from build123d import *

# Parameters (mm, degrees)
SKETCH_1_R               = 9
SKETCH_1_R_2             = 29.6
SKETCH_1_R_3             = 1.5
EXTRUDE_1_DEPTH          = 3
CUT_EXTRUDE_1_DEPTH      = 287.481238478
CUT_EXTRUDE_1_DEPTH_BACK = 287.481238478
SKETCH_2_R               = 1.25
CUT_EXTRUDE_2_DEPTH      = 287.481238478
CUT_EXTRUDE_2_DEPTH_BACK = 287.481238478
CUT_EXTRUDE_3_DEPTH      = 287.481238478
CUT_EXTRUDE_3_DEPTH_BACK = 287.481238478
SKETCH_4_R               = 1.5


with BuildPart() as part:
    # 草图1 → 凸台-拉伸1 (new body)
    with BuildSketch(Plane(origin=(0, 0, 0), x_dir=(1, 0, 0), z_dir=(0, 1, 0))):
        with BuildLine():
            Line((71.271215686, 30), (163.728784314, 30))
            ThreePointArc((163.728784314, 30), (189.096168452, 33.068787794), (213, 42.09809972))
            ThreePointArc((213, 42.09809972), (282.5, 0), (213, -42.09809972))
            ThreePointArc((213, -42.09809972), (189.096168452, -33.068787794), (163.728784314, -30))
            Line((163.728784314, -30), (71.271215686, -30))
            ThreePointArc((71.271215686, -30), (45.903831548, -33.068787794), (22, -42.09809972))
            ThreePointArc((22, -42.09809972), (-47.5, 0), (22, 42.09809972))
            ThreePointArc((22, 42.09809972), (45.903831548, 33.068787794), (71.271215686, 30))
        make_face()
        with Locations(Location((0, 0, 0), (0, 0, 270))):
            Circle(SKETCH_1_R, mode=Mode.SUBTRACT)
        with Locations(Location((235, 0, 0), (0, 0, 270))):
            Circle(SKETCH_1_R_2, mode=Mode.SUBTRACT)
        with Locations(Location((218.735954124, 39.264880132, 0), (0, 0, 270))):
            Circle(SKETCH_1_R_3, mode=Mode.SUBTRACT)
        with Locations(Location((251.264045876, 39.264880132, 0), (0, 0, 270))):
            Circle(SKETCH_1_R_3, mode=Mode.SUBTRACT)
        with Locations(Location((274.264880132, 16.264045876, 0), (0, 0, 270))):
            Circle(SKETCH_1_R_3, mode=Mode.SUBTRACT)
        with Locations(Location((195.735119868, 16.264045876, 0), (0, 0, 270))):
            Circle(SKETCH_1_R_3, mode=Mode.SUBTRACT)
        with Locations(Location((195.735119868, -16.264045876, 0), (0, 0, 270))):
            Circle(SKETCH_1_R_3, mode=Mode.SUBTRACT)
        with Locations(Location((274.264880132, -16.264045876, 0), (0, 0, 270))):
            Circle(SKETCH_1_R_3, mode=Mode.SUBTRACT)
        with Locations(Location((251.264045876, -39.264880132, 0), (0, 0, 270))):
            Circle(SKETCH_1_R_3, mode=Mode.SUBTRACT)
        with Locations(Location((218.735954124, -39.264880132, 0), (0, 0, 270))):
            Circle(SKETCH_1_R_3, mode=Mode.SUBTRACT)
        with Locations(Location((-16.264045876, 39.264880132, 0), (0, 0, 270))):
            Circle(SKETCH_1_R_3, mode=Mode.SUBTRACT)
        with Locations(Location((16.264045876, 39.264880132, 0), (0, 0, 270))):
            Circle(SKETCH_1_R_3, mode=Mode.SUBTRACT)
        with Locations(Location((39.264880132, 16.264045876, 0), (0, 0, 270))):
            Circle(SKETCH_1_R_3, mode=Mode.SUBTRACT)
        with Locations(Location((39.264880132, -16.264045876, 0), (0, 0, 270))):
            Circle(SKETCH_1_R_3, mode=Mode.SUBTRACT)
        with Locations(Location((16.264045876, -39.264880132, 0), (0, 0, 270))):
            Circle(SKETCH_1_R_3, mode=Mode.SUBTRACT)
        with Locations(Location((-16.264045876, -39.264880132, 0), (0, 0, 270))):
            Circle(SKETCH_1_R_3, mode=Mode.SUBTRACT)
        with Locations(Location((-39.264880132, -16.264045876, 0), (0, 0, 270))):
            Circle(SKETCH_1_R_3, mode=Mode.SUBTRACT)
        with Locations(Location((-39.264880132, 16.264045876, 0), (0, 0, 270))):
            Circle(SKETCH_1_R_3, mode=Mode.SUBTRACT)
        with Locations(Location((-6.783865663, 11.75, 0), (0, 0, 270))):
            Circle(SKETCH_1_R_3, mode=Mode.SUBTRACT)
        with Locations(Location((6.783865663, 11.75, 0), (0, 0, 270))):
            Circle(SKETCH_1_R_3, mode=Mode.SUBTRACT)
        with Locations(Location((13.567731326, 0, 0), (0, 0, 270))):
            Circle(SKETCH_1_R_3, mode=Mode.SUBTRACT)
        with Locations(Location((6.783865663, -11.75, 0), (0, 0, 270))):
            Circle(SKETCH_1_R_3, mode=Mode.SUBTRACT)
        with Locations(Location((-13.567731326, 0, 0), (0, 0, 270))):
            Circle(SKETCH_1_R_3, mode=Mode.SUBTRACT)
        with Locations(Location((-6.783865663, -11.75, 0), (0, 0, 270))):
            Circle(SKETCH_1_R_3, mode=Mode.SUBTRACT)
    extrude(amount=EXTRUDE_1_DEPTH)

    # 草图2 → 切除-拉伸1 (cut, two sides: drawn at the far end of the back side and taken through both)
    with BuildSketch(Plane(origin=(0, 3, 0), x_dir=(1, 0, 0), z_dir=(0, 1, 0)).offset(-CUT_EXTRUDE_1_DEPTH_BACK)):
        with Locations(Location((93.271215686, 25, 0), (0, 0, 270))):
            Circle(SKETCH_2_R)
        with Locations(Location((141.728784314, 25, 0), (0, 0, 270))):
            Circle(SKETCH_2_R)
        with Locations(Location((190.288457303, 28.213023457, 0), (0, 0, 270))):
            Circle(SKETCH_2_R)
        with Locations(Location((44.711542697, 28.213023457, 0), (0, 0, 270))):
            Circle(SKETCH_2_R)
        with Locations(Location((44.711542697, -28.213023457, 0), (0, 0, 270))):
            Circle(SKETCH_2_R)
        with Locations(Location((93.271215686, -25, 0), (0, 0, 270))):
            Circle(SKETCH_2_R)
        with Locations(Location((190.288457303, -28.213023457, 0), (0, 0, 270))):
            Circle(SKETCH_2_R)
        with Locations(Location((141.728784314, -25, 0), (0, 0, 270))):
            Circle(SKETCH_2_R)
    extrude(amount=CUT_EXTRUDE_1_DEPTH + CUT_EXTRUDE_1_DEPTH_BACK, mode=Mode.SUBTRACT)

    # 草图3 → 切除-拉伸2 (cut, two sides: drawn at the far end of the back side and taken through both)
    with BuildSketch(Plane(origin=(0, 3, 0), x_dir=(1, 0, 0), z_dir=(0, 1, 0)).offset(-CUT_EXTRUDE_2_DEPTH_BACK)):
        with BuildLine():
            ThreePointArc((-12.848523388, -12.960630646), (-9.125, -15.804963619), (-4.799973695, -17.607462978))
            ThreePointArc((-4.799973695, -17.607462978), (-2.52132569, -19.251580515), (-1.886243278, -21.988737715))
            Line((-1.886243278, -21.988737715), (-3.494651309, -34.205809627))
            ThreePointArc((-3.494651309, -34.205809627), (-5.165797392, -36.960083611), (-8.325408233, -37.589061943))
            ThreePointArc((-8.325408233, -37.589061943), (-19.25, -33.341978046), (-28.390378431, -26.004545998))
            ThreePointArc((-28.390378431, -26.004545998), (-29.425472637, -22.953753578), (-27.875774439, -20.129361624))
            Line((-27.875774439, -20.129361624), (-18.099683819, -12.627903454))
            ThreePointArc((-18.099683819, -12.627903454), (-15.411694944, -11.809322357), (-12.848523388, -12.960630646))
        make_face()
        with BuildLine():
            ThreePointArc((-17.648497083, 4.646832332), (-18.25, 0), (-17.648497083, -4.646832332))
            ThreePointArc((-17.648497083, -4.646832332), (-17.933020634, -7.442258159), (-19.985927097, -9.360834261))
            Line((-19.985927097, -9.360834261), (-31.370425748, -14.076448003))
            ThreePointArc((-31.370425748, -14.076448003), (-34.591270029, -14.006330033), (-36.715786664, -11.584515945))
            ThreePointArc((-36.715786664, -11.584515945), (-38.5, 0), (-36.715786664, 11.584515945))
            ThreePointArc((-36.715786664, 11.584515945), (-34.591270029, 14.006330033), (-31.370425748, 14.076448003))
            Line((-31.370425748, 14.076448003), (-19.985927097, 9.360834261))
            ThreePointArc((-19.985927097, 9.360834261), (-17.933020634, 7.442258159), (-17.648497083, 4.646832332))
        make_face()
        with BuildLine():
            ThreePointArc((-4.799973695, 17.607462978), (-9.125, 15.804963619), (-12.848523388, 12.960630646))
            ThreePointArc((-12.848523388, 12.960630646), (-15.411694944, 11.809322357), (-18.099683819, 12.627903454))
            Line((-18.099683819, 12.627903454), (-27.875774439, 20.129361624))
            ThreePointArc((-27.875774439, 20.129361624), (-29.425472637, 22.953753578), (-28.390378431, 26.004545998))
            ThreePointArc((-28.390378431, 26.004545998), (-19.25, 33.341978046), (-8.325408233, 37.589061943))
            ThreePointArc((-8.325408233, 37.589061943), (-5.165797392, 36.960083611), (-3.494651309, 34.205809627))
            Line((-3.494651309, 34.205809627), (-1.886243278, 21.988737715))
            ThreePointArc((-1.886243278, 21.988737715), (-2.52132569, 19.251580515), (-4.799973695, 17.607462978))
        make_face()
        with BuildLine():
            ThreePointArc((12.848523388, 12.960630646), (9.125, 15.804963619), (4.799973695, 17.607462978))
            ThreePointArc((4.799973695, 17.607462978), (2.52132569, 19.251580515), (1.886243278, 21.988737715))
            Line((1.886243278, 21.988737715), (3.494651309, 34.205809627))
            ThreePointArc((3.494651309, 34.205809627), (5.165797392, 36.960083611), (8.325408233, 37.589061943))
            ThreePointArc((8.325408233, 37.589061943), (19.25, 33.341978046), (28.390378431, 26.004545998))
            ThreePointArc((28.390378431, 26.004545998), (29.425472637, 22.953753578), (27.875774439, 20.129361624))
            Line((27.875774439, 20.129361624), (18.099683819, 12.627903454))
            ThreePointArc((18.099683819, 12.627903454), (15.411694944, 11.809322357), (12.848523388, 12.960630646))
        make_face()
        with BuildLine():
            ThreePointArc((17.648497083, -4.646832332), (18.25, 0), (17.648497083, 4.646832332))
            ThreePointArc((17.648497083, 4.646832332), (17.933020634, 7.442258159), (19.985927097, 9.360834261))
            Line((19.985927097, 9.360834261), (31.370425748, 14.076448003))
            ThreePointArc((31.370425748, 14.076448003), (34.591270029, 14.006330033), (36.715786664, 11.584515945))
            ThreePointArc((36.715786664, 11.584515945), (38.5, 0), (36.715786664, -11.584515945))
            ThreePointArc((36.715786664, -11.584515945), (34.591270029, -14.006330033), (31.370425748, -14.076448003))
            Line((31.370425748, -14.076448003), (19.985927097, -9.360834261))
            ThreePointArc((19.985927097, -9.360834261), (17.933020634, -7.442258159), (17.648497083, -4.646832332))
        make_face()
        with BuildLine():
            ThreePointArc((4.799973695, -17.607462978), (9.125, -15.804963619), (12.848523388, -12.960630646))
            ThreePointArc((12.848523388, -12.960630646), (15.411694944, -11.809322357), (18.099683819, -12.627903454))
            Line((18.099683819, -12.627903454), (27.875774439, -20.129361624))
            ThreePointArc((27.875774439, -20.129361624), (29.425472637, -22.953753578), (28.390378431, -26.004545998))
            ThreePointArc((28.390378431, -26.004545998), (19.25, -33.341978046), (8.325408233, -37.589061943))
            ThreePointArc((8.325408233, -37.589061943), (5.165797392, -36.960083611), (3.494651309, -34.205809627))
            Line((3.494651309, -34.205809627), (1.886243278, -21.988737715))
            ThreePointArc((1.886243278, -21.988737715), (2.52132569, -19.251580515), (4.799973695, -17.607462978))
        make_face()
    extrude(amount=CUT_EXTRUDE_2_DEPTH + CUT_EXTRUDE_2_DEPTH_BACK, mode=Mode.SUBTRACT)

    # 草图4 → 切除-拉伸3 (cut, two sides: drawn at the far end of the back side and taken through both)
    with BuildSketch(Plane(origin=(0, 3, 0), x_dir=(1, 0, 0), z_dir=(0, 1, 0)).offset(-CUT_EXTRUDE_3_DEPTH_BACK)):
        with Locations(Location((68.264880132, 16.264045876, 0), (0, 0, 270))):
            Circle(SKETCH_4_R)
        with Locations(Location((110.264880132, 16.264045876, 0), (0, 0, 270))):
            Circle(SKETCH_4_R)
        with Locations(Location((152.264880132, 16.264045876, 0), (0, 0, 270))):
            Circle(SKETCH_4_R)
        with Locations(Location((181.264880132, 16.264045876, 0), (0, 0, 270))):
            Circle(SKETCH_4_R)
        with Locations(Location((68.264880132, -16.264045876, 0), (0, 0, 270))):
            Circle(SKETCH_4_R)
        with Locations(Location((110.264880132, -16.264045876, 0), (0, 0, 270))):
            Circle(SKETCH_4_R)
        with Locations(Location((152.264880132, -16.264045876, 0), (0, 0, 270))):
            Circle(SKETCH_4_R)
        with Locations(Location((181.264880132, -16.264045876, 0), (0, 0, 270))):
            Circle(SKETCH_4_R)
    extrude(amount=CUT_EXTRUDE_3_DEPTH + CUT_EXTRUDE_3_DEPTH_BACK, mode=Mode.SUBTRACT)


solid = part.part
Check sheet for the modelled part. Datum: model origin and axes. Units: mm. A direction names the side the tool comes from. Round coordinates to 2 decimals unless told otherwise and drop trailing zeros. Loops run counter-clockwise (first coordinate to the right, second up) from the corner with the lowest first, then second, coordinate; pieces in that order, holes last.
1. Sectioned sample at D-D on x = 186. Record the boundary of the cut face in (y, z).
2. Sectioned sample at B-B on y = 1.7. Give the number of separate pieces and of enclosed holes in the cut face, and give its area (3 significant figures).
3. Gauge pin test, flat ends, axial feed: pin 1 Ø2.5 at (x, z) = (110.26, -16.26) entering from -Y; pin 2 Ø8 at (x, z) = (245, 31) entering from -Y; pin 3 Ø1 at (x, y) = (233, 2) entering from -Z; pin 4 Ø1 at (y, z) = (0.5, 36.5) entering from +X. Record the tip position at first contact, or that the pin passes through.
4. Sectioned sample at C-C on x = 129. Record the boundary of the cut face in (y, z).
5. Set-up check for faces 4 (the cylindrical face through (188.748, 1.479, -32.984)), 5 (the flat face through (120, 3, -1)), 6 (the cylindrical face through (46.252, 1.479, 32.984)), 7 (the flat face through (22.919, 1.479, 16.326)): record each of +Z, -Z, +X, -X, +Y, -Y from which the full face is reachable in a straight line by a thin tool's end or side.
6. Sectioned sample at A-A on x = 235. Record the boundary of the cut face in (y, z).
7. Mould release check, pull along Z, two halves, no side actions. Record for faces 1 (the cylindrical face through (189.444, 1.479, 33.155)), 2 (the cylindrical face through (19.107, 1.479, -33.424)), 3 (the flat face through (120, 0, -1)): released by +Z, released by -Z, zero draft, split by the parting line, or undercut.
8. Scan lines: probe 1 along X at (y, z) = (1.15, -19); probe 2 along Z at (x, y) = (218, 0.2); probe 3 along X at (y, z) = (0.7, 4). Record each from-to range of solid material in increasing order.
Recorded:
1. outline: (0, -32.36) - (3, -32.36) - (3, 32.36) - (0, 32.36) - close
2. separate pieces: 1
2. enclosed holes: 46
2. area: 17,200 mm2
3. pin 1: passes through
3. pin 2: stops at y = 0
3. pin 3: stops at z = -47.48
3. pin 4: stops at x = 265.99
4. outline: (0, -30) - (3, -30) - (3, 30) - (0, 30) - close
5. face 4: -Z, +Y, -Y
5. face 5: +Z, -Z, +X, -X, +Y
5. face 6: +Z, +Y, -Y
5. face 7: +Y, -Y
6. outline: (0, -47.5) - (3, -47.5) - (3, -29.6) - (0, -29.6) - close; (0, 29.6) - (3, 29.6) - (3, 47.5) - (0, 47.5) - close
7. face 1: released by +Z
7. face 2: undercut
7. face 3: zero draft
8. probe 1: x = -43.53 to -26.4, -2.7 to 2.7, 26.4 to 212.3, 257.7 to 278.53
8. probe 2: z = -44.35 to -40.57, -37.96 to -24.23, 24.23 to 37.96, 40.57 to 44.35
8. probe 3: x = -47.33 to -38.29, -17.81 to -8.06, 8.06 to 17.81, 38.29 to 205.67, 264.33 to 282.33
